```python
from build123d import *

# Parameters (mm, degrees)
BASELINE_BODY_DEPTH   = 7.5
SKETCH3_R             = 5
CUT_EXTRUDE1_DEPTH    = 159.837149307
SKETCH4_R             = 25
BOSS_EXTRUDE2_DEPTH   = 15
SKETCH5_R             = 12
CUT_EXTRUDE2_DEPTH    = 161.947941894
SKETCH6_R             = 13
CUT_EXTRUDE3_DEPTH    = 9
CUT_EXTRUDE4_START    = -9
SKETCH7_R             = 13
CUT_EXTRUDE4_DEPTH    = 9
M4_TAPPED_HOLE6_D     = 3.3
M4_TAPPED_HOLE6_DEPTH = 9
M4_TAPPED_HOLE6_TIP   = 0.991420021
M4_TAPPED_HOLE8_D     = 3.3
M4_TAPPED_HOLE8_DEPTH = 9
M4_TAPPED_HOLE8_TIP   = 0.991420021


with BuildPart() as part:
    # Rocker_Profile → Baseline_Body (new, symmetric)
    with BuildSketch(Plane.XY):
        with BuildLine():
            Line((-97.302083333, -24.966068553), (-1.5625, -29.959282264))
            ThreePointArc((-1.5625, -29.959282264), (17.206458335, -24.57514581), (28.686326507, -8.780357142))
            Line((28.686326507, -8.780357142), (52.641312178, 69.483035715))
            ThreePointArc((52.641312178, 69.483035715), (44.023831603, 96.580885487), (15.628732451, 98.088458997))
            Line((15.628732451, 98.088458997), (-109.107307638, 21.288458997))
            ThreePointArc((-109.107307638, 21.288458997), (-120.2235003, -6.182397046), (-97.302083333, -24.966068553))
        make_face()
    extrude(amount=BASELINE_BODY_DEPTH, both=True)

    # Sketch3 → Cut-Extrude1 (cut, through all)
    with BuildSketch(Plane.XY.offset(7.5)):
        with Locations((-96, 0)):
            Circle(SKETCH3_R)
        with Locations((28.736040089, 76.8)):
            Circle(SKETCH3_R)
    extrude(amount=-CUT_EXTRUDE1_DEPTH, mode=Mode.SUBTRACT)

    # Sketch4 → Boss-Extrude2 (add, symmetric)
    with BuildSketch(Plane.XY):
        Circle(SKETCH4_R)
    extrude(amount=BOSS_EXTRUDE2_DEPTH, both=True)

    # Sketch5 → Cut-Extrude2 (cut, through all)
    with BuildSketch(Plane.XY.offset(15)):
        Circle(SKETCH5_R)
    extrude(amount=-CUT_EXTRUDE2_DEPTH, mode=Mode.SUBTRACT)

    # Sketch6 → Cut-Extrude3 (cut)
    with BuildSketch(Plane.XY.offset(15)):
        Circle(SKETCH6_R)
    extrude(amount=-CUT_EXTRUDE3_DEPTH, mode=Mode.SUBTRACT)

    # Sketch7 → Cut-Extrude4 (cut)
    with BuildSketch(Plane(origin=(0, 0, -15), x_dir=(-1, 0, 0), z_dir=(0, 0, -1)).offset(CUT_EXTRUDE4_START)):
        with Locations(Location((0, 0, 0), (0, 0, 180))):
            Circle(SKETCH7_R)
    extrude(amount=CUT_EXTRUDE4_DEPTH, mode=Mode.SUBTRACT)

    # M4 Tapped Hole6
    with Locations(Plane.XY.offset(15)):
        with Locations((-15.588457268, -9), (0, 18), (15.588457268, -9)):
            Hole(M4_TAPPED_HOLE6_D / 2, depth=M4_TAPPED_HOLE6_DEPTH)
            with Locations((0, 0, -(M4_TAPPED_HOLE6_DEPTH + M4_TAPPED_HOLE6_TIP / 2))):  # 118° drill point
                Cone(0, M4_TAPPED_HOLE6_D / 2, M4_TAPPED_HOLE6_TIP, mode=Mode.SUBTRACT)

    # M4 Tapped Hole8
    with Locations(Plane(origin=(0, 0, -15), x_dir=(-1, 0, 0), z_dir=(0, 0, -1))):
        with Locations((-15.588457268, -9), (0, 18), (15.585467422, -8.998273811)):
            Hole(M4_TAPPED_HOLE8_D / 2, depth=M4_TAPPED_HOLE8_DEPTH)
            with Locations((0, 0, -(M4_TAPPED_HOLE8_DEPTH + M4_TAPPED_HOLE8_TIP / 2))):  # 118° drill point
                Cone(0, M4_TAPPED_HOLE8_D / 2, M4_TAPPED_HOLE8_TIP, mode=Mode.SUBTRACT)


solid = part.part
```
Model file for the job. Use its own axes, mm. A direction names the side the tool comes from. Coordinates: 2 decimals unless noted, no trailing zeros. Write each loop counter-clockwise with the first axis right and the second up, starting at its lowest first coordinate (ties: lowest second). Pieces come first, ordered by that corner, then holes. Notation, with made-up numbers: (76.25, -21) - (117.25, -21) arc R20 cw to (117.25, 12) - close; hole circle Ø4 at (-15, 29). An arc over 180 degrees is marked (long way). One line per item, written item: value. Start each with the question number.
1. Slice it at C-C (x = -38). Write the cut outline in (y, z).
2. Slice it at D-D (y = 32.5). Write the cut outline in (x, z), plus the area to 3 significant figures.
3. Flat gauge pins, fed straight in: pin 1 (3 mm diameter, centred on x = 26.5, z = 2.5, fed in from -Y); pin 2 (21 mm diameter, centred on x = 0, y = 0, fed in from +Z); pin 3 (6 mm diameter, centred on y = 18.5, z = 7, fed in from +X); pin 4 (6 mm diameter, centred on y = 27.5, z = 7, fed in from +X). Where does each tip first touch, or does it go through?
4. Slice it at B-B (y = 76.8). Write the cut outline in (x, z).
5. Probe line 1 (Y direction, x = 0, z = -2.5); line 2 (Z direction, x = -44, y = 29); line 3 (X direction, y = -9, z = 12). List the from-to ranges inside material, lowest first. Write a range as from..to.
6. Mould opens along Y. For faces 1 (the flat face through (40.496, 29.803, 0.105)), 2 (the cylindrical face through (23.846, 7.509, 11.302)), 3 (the flat face through (9, -9, 6)) say: released by +Y, released by -Y, zero draft, split by the parting line, or undercut.
7. Slice it at A-A (z = 11.5). Write the cut outline in (x, y), plus the area to 3 significant figures.
8. Tool access for faces 4 (the cylindrical face through (-10.316, -7.91, 10.563)), 5 (the cylindrical face through (-91.381, -1.915, 0.105)), 6 (the cylindrical face through (23.846, 7.509, -11.198)): list every direction of +Z, -Z, +X, -X, +Y, -Y with a clear straight run to the whole face (end or side of a thin tool).
Answers below:
1. outline: (-28.06, -7.5) - (65.07, -7.5) - (65.07, 7.5) - (-28.06, 7.5) - close
2. outline: (-90.9, -7.5) - (41.32, -7.5) - (41.32, 7.5) - (-90.9, 7.5) - close
2. area: 1,980 mm^2
3. pin 1: stops at y = -16.58
3. pin 2: passes through
3. pin 3: stops at x = 37.95
3. pin 4: stops at x = 40.71
4. outline: (-18.95, -7.5) - (23.74, -7.5) - (23.74, 7.5) - (-18.95, 7.5) - close; (33.74, -7.5) - (53.74, -7.5) - (53.74, 7.5) - (33.74, 7.5) - close
5. line 1: y = -30..-12, 12..88.47
5. line 2: z = -7.5..7.5
5. line 3: x = -23.32..-17.24, -13.94..-9.38, 9.38..13.94, 17.24..23.32
6. face 1: released by -Y
6. face 2: split by the parting line
6. face 3: undercut
7. outline: circle Ø50 at (0, 0); hole circle Ø3.3 at (-15.59, -9); hole circle Ø26 at (0, 0); hole circle Ø3.3 at (0, 18); hole circle Ø3.3 at (15.59, -9)
7. area: 1,410 mm^2
8. face 4: +Z
8. face 5: +Z, -Z
8. face 6: -Z
